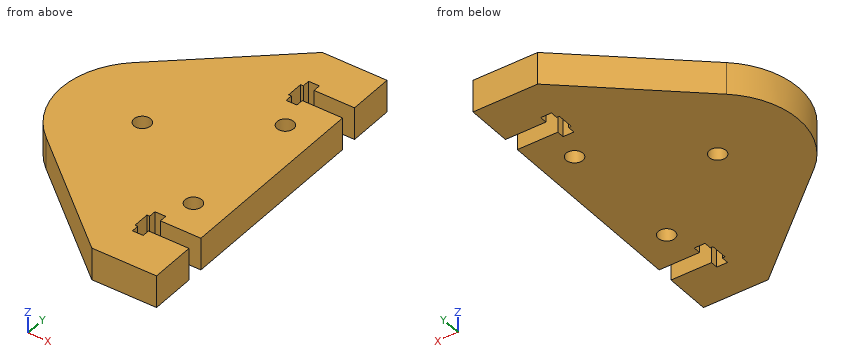
from build123d import *

# Parameters (mm, degrees)
DODANIE_WYCI_GNI_CIE1_DEPTH = 6
SZKIC2_R                    = 1.55
WYTNIJ_WYCI_GNI_CIE1_DEPTH  = 6
WYTNIJ_WYCI_GNI_CIE2_DEPTH  = 6
SZYK_LINIOWY1_COUNT         = 2
SZYK_LINIOWY1_PITCH         = 40
SZKIC4_R                    = 1.55
WYTNIJ_WYCI_GNI_CIE3_DEPTH  = 6


with BuildPart() as part:
    # Szkic1 → Dodanie-wyciągnięcie1 (new body)
    with BuildSketch(Plane.XY):
        with BuildLine():
            Line((-455.064585695, -113.955768861), (-476.813799507, -95.355454386))
            ThreePointArc((-476.813799507, -95.355454386), (-482.064585695, -83.955768861), (-476.813799507, -72.556083337))
            Line((-476.813799507, -72.556083337), (-455.064585695, -53.955768861))
            Line((-455.064585695, -53.955768861), (-443.064585695, -53.955768861))
            Line((-443.064585695, -53.955768861), (-443.064585695, -113.955768861))
            Line((-443.064585695, -113.955768861), (-455.064585695, -113.955768861))
        make_face()
    extrude(amount=DODANIE_WYCI_GNI_CIE1_DEPTH)

    # Szkic2 → Wytnij-wyciągnięcie1 (cut)
    with BuildSketch(Plane.XY.offset(6)):
        with Locations((-467.064585695, -83.955768861)):
            Circle(SZKIC2_R)
    extrude(amount=-WYTNIJ_WYCI_GNI_CIE1_DEPTH, mode=Mode.SUBTRACT)

    # Szkic3 → Wytnij-wyciągnięcie2 (cut)
    with BuildSketch(Plane(origin=(0, 0, 0), x_dir=(-1, 0, 0), z_dir=(0, 0, -1))):
        Polygon((443.064585695, -105.505768861), (450.564585695, -105.505768861), (450.564585695, -106.880768861), (452.564585695, -106.880768861), (452.564585695, -105.505768861), (453.064585695, -105.505768861), (453.064585695, -102.405768861), (452.564585695, -102.405768861), (452.564585695, -101.030768861), (450.564585695, -101.030768861), (450.564585695, -102.405768861), (443.064585695, -102.405768861), align=None)
    wytnij_wyci_gni_cie2 = extrude(amount=-WYTNIJ_WYCI_GNI_CIE2_DEPTH, mode=Mode.SUBTRACT)

    # Szyk liniowy1: Wytnij-wyciągnięcie2 ×2
    with Locations(*[(0, i * SZYK_LINIOWY1_PITCH, 0) for i in range(1, SZYK_LINIOWY1_COUNT)]):
        add(wytnij_wyci_gni_cie2, mode=Mode.SUBTRACT)

    # Szkic4 → Wytnij-wyciągnięcie3 (cut)
    with BuildSketch(Plane(origin=(0, 0, 0), x_dir=(-1, 0, 0), z_dir=(0, 0, -1))):
        with Locations((449.064585017, -95.936775964)):
            Circle(SZKIC4_R)
        with Locations((449.064585017, -71.970769345)):
            Circle(SZKIC4_R)
    extrude(amount=-WYTNIJ_WYCI_GNI_CIE3_DEPTH, mode=Mode.SUBTRACT)


solid = part.part
Geometry: final body of the model. Coordinates: model frame, mm. Give positions to 0.01 mm unless a question says otherwise; leave off trailing zeros. Loops run counter-clockwise (first coordinate to the right, second up) from the corner with the lowest first, then second, coordinate; pieces in that order, holes last. Notation, with made-up numbers: M 35.25,-31 L 71.25,-31 A7 ccw 71.25,-19 Z; hole C 66,77 d6. An arc over 180 degrees is marked long. Put each result on its own line as item: value.
1) Cut plane B-B, the plane z = 0.75. Give the number of separate pieces and of enclosed holes in the cut face, plus the area to 3 significant figures.
Computed values:
separate pieces: 1
enclosed holes: 3
area: 1,610 mm^2
2) Cut plane C-C, the plane x = -474. Return the cut outline in (y, z), plus the area to 3 significant figures.
Computed values:
outline: M -97.76,0 L -70.15,0 L -70.15,6 L -97.76,6 Z
area: 166 mm^2
3) Material intervals for L1, parallel to Y at x = -452.5, z = 4.4; L2, parallel to Y at x = -446.5, z = 0.45; L3, parallel to Y at x = -449.5, z = 0.8, sorted ascending. Write a range as from..to.
Computed values:
L1: y = -113.96..-106.88, -101.03..-66.88, -61.03..-53.96
L2: y = -113.96..-105.51, -102.41..-65.51, -62.41..-53.96
L3: y = -113.96..-105.51, -102.41..-97.42, -94.45..-73.46, -70.48..-65.51, -62.41..-53.96
4) Cut plane D-D, the plane y = -90.5. Return the cut outline in (x, z).
Computed values:
outline: M -480.56,0 L -443.06,0 L -443.06,6 L -480.56,6 Z
5) Cut plane A-A, the plane x = -467. Return the cut outline in (y, z).
Computed values:
outline: M -103.75,0 L -85.5,0 L -85.5,6 L -103.75,6 Z; M -82.41,0 L -64.16,0 L -64.16,6 L -82.41,6 Z
6) First-contact query: P1, Ø2.5, axis at x = -467.06, y = -83.96, coming from the +Z side; P2, Ø1.5, axis at x = -464, z = 2, coming from the -Y side; P3, Ø1, axis at x = -471.5, z = 5, coming from the -Y side; P4, Ø1, axis at y = -86.5, z = 5.5, coming from the -X side. Flat tips, straight axial feed; report the tip coordinate or a pass-through.
Computed values:
P1: passes through
P2: stops at y = -106.96
P3: stops at y = -100.33
P4: stops at x = -481.92
